```python
from build123d import *

# Parameters (mm, degrees)
F0_R     = 6
F0_R_2   = 1.75
F4_DEPTH = 1
F5_R     = 0.5


with BuildPart() as f3:
    # F2 (on Front) → F3 (revolve)
    with BuildSketch(Plane.XZ):
        Polygon((1.75, 0), (2.5, 0), (2.5, 5), (2, 5), align=None)
    revolve(axis=Axis((0, 0, 2), (0, 0, 1)))

    # F0 (on Top) → F4 (join)
    with BuildSketch(Plane.XY):
        Circle(F0_R)
        Circle(F0_R_2, mode=Mode.SUBTRACT)
    extrude(amount=F4_DEPTH)

    # F5
    f5_edges = [f3.edges().sort_by_distance(p)[0] for p in [
        (-2.5, 0, 1),
    ]]
    fillet(f5_edges, radius=F5_R)


solid = f3.part
```
Check sheet for the modelled part. Datum: model origin and axes. Units: mm. A direction names the side the tool comes from. Round coordinates to 2 decimals unless told otherwise and drop trailing zeros. Loops run counter-clockwise (first coordinate to the right, second up) from the corner with the lowest first, then second, coordinate; pieces in that order, holes last. Notation, with made-up numbers: (-35.75, 68.25) -> (21.25, 68.25) arc R22 cw to (21.25, 99.25) -> close; hole circle Ø7 at (83, 32.5). An arc over 180 degrees is marked (long way). Write item = value, one per line. Start each with the question number.
1) Sectioned sample at C-C, the plane z = 1.25. Record the cut outline in (x, y) (1 decimal), plus the area to 3 significant figures.
2) Thickness scan on probe 1 along Y at (x, z) = (0, 0.45); probe 2 along Z at (x, y) = (1, -3.5); probe 3 along Y at (x, z) = (-1.75, 4.1). Record the ranges inside material, lowest first.
3) Release check for a two-part mould opening along Y. For faces 3 (the cylindrical face through (-5.994, 0.264, 0.493)), 4 (the cylindrical face through (1.617, -0.67, 0.493)), 5 (the flat face through (-1, 2, 5)) record: released by +Y, released by -Y, zero draft, split by the parting line, or undercut.
4) Gauge pin test, flat ends, axial feed: pin 1 Ø2 at (x, z) = (2, 3.5) entering from +Y; pin 2 Ø1 at (x, y) = (2, -3.5) entering from +Z; pin 3 Ø1.5 at (x, z) = (-2, 1.5) entering from +Y. Record the tip position at first contact, or that the pin passes through.
5) Sectioned sample at A-A, the plane y = 0. Record the cut outline in (x, z).
6) Sectioned sample at D-D, the plane x = -3.5. Record the cut outline in (y, z), plus the area to 3 significant figures.
7) Set-up check for faces 1 (the cylindrical face through (-0.54, -2.44, 3.27)), 2 (the flat face through (-1.4, 1.4, 0)): record each of +Z, -Z, +X, -X, +Y, -Y from which the full face is reachable in a straight line by a thin tool's end or side.
Results are:
q1.outline = circle Ø5.1 at (0, 0); hole circle Ø3.6 at (0, 0)
q1.area = 10.4 mm^2
q2.probe_1 = -6 to -1.75, 1.75 to 6
q2.probe_2 = 0 to 1
q2.probe_3 = -1.79 to -0.87, 0.87 to 1.79
q3.face_3 = split by the parting line
q3.face_4 = undercut
q3.face_5 = zero draft
q4.pin_1 = 2.29
q4.pin_2 = 1
q4.pin_3 = 5.82
q5.outline = (-6, 0) -> (-1.75, 0) -> (-1.75, 1) -> (-1.8, 1) -> (-2, 5) -> (-2.5, 5) -> (-2.5, 1.5) arc R0.5 cw to (-3, 1) -> (-6, 1) -> close; (1.75, 0) -> (6, 0) -> (6, 1) -> (3, 1) arc R0.5 cw to (2.5, 1.5) -> (2.5, 5) -> (2, 5) -> (1.8, 1) -> (1.75, 1) -> close
q6.outline = (-4.87, 0) -> (4.87, 0) -> (4.87, 1) -> (-4.87, 1) -> close
q6.area = 9.75 mm^2
q7.face_1 = +Z
q7.face_2 = -Z, +X, -X, +Y, -Y
